from build123d import *

# Parameters (mm, degrees)
SKETCH_2_R      = 2
EXTRUDE_1_DEPTH = 2.5


with BuildPart() as part:
    # 草圖2 → 填料-伸長1 (new, symmetric)
    with BuildSketch(Plane.XY):
        with BuildLine():
            Line((7.226190238, -41.651673377), (4.413452329, 1.473554067))
            ThreePointArc((4.413452329, 1.473554067), (1.735862232, 4.991257537), (-2.546669656, 3.894149036))
            Line((-2.546669656, 3.894149036), (-41.492870765, -39.231078407))
            ThreePointArc((-41.492870765, -39.231078407), (-42.179656235, -43.536244411), (-38.524267862, -45.912010486))
            Line((-38.524267862, -45.912010486), (3.234671155, -45.912010486))
            ThreePointArc((3.234671155, -45.912010486), (6.153690549, -44.64684609), (7.226190238, -41.651673377))
        make_face()
        Circle(SKETCH_2_R, mode=Mode.SUBTRACT)
        with Locations((2.700997506, -41.412010486)):
            Circle(SKETCH_2_R, mode=Mode.SUBTRACT)
        with Locations((-37.399002494, -41.412010486)):
            Circle(SKETCH_2_R, mode=Mode.SUBTRACT)
    extrude(amount=EXTRUDE_1_DEPTH, both=True)


solid = part.part
Source: CAD feature listing. Evaluate the final solid. Frame: model axes, mm. Give positions to 0.01 mm unless a question says otherwise; leave off trailing zeros. Write each loop counter-clockwise with the first axis right and the second up, starting at its lowest first coordinate (ties: lowest second). Pieces come first, ordered by that corner, then holes. Notation, with made-up numbers: (57.25, 87.25) -> (106.25, 87.25) arc R32 cw to (106.25, 119.25) -> close; hole circle Ø6 at (22.5, 20.5). An arc over 180 degrees is marked (long way). Return JSON: item names as keys, results as strings. Group by question number.
1. Section C-C, the plane z = 1.2. Output: boundary loops of the cut face in (x, y).
2. Section D-D, the plane y = -34.5. Output: boundary loops of the cut face in (x, z).
3. Section B-B, the plane y = 0. Output: boundary loops of the cut face in (x, z).
4. Pin query (flat end, axial travel): pin 1 Ø3.5 at (x, y) = (-37.4, -41.41) entering from +Z; pin 2 Ø1.5 at (y, z) = (-27, -1) entering from +X. Return the tip coordinate at first contact, or that it passes through.
5. Material intervals for line 1 (Y direction, x = 3.5, z = -2.3); line 2 (Y direction, x = -39, z = -1.1); line 3 (X direction, y = -18, z = 1.15), sorted ascending. Write a range as from..to.
6. Section A-A, the plane x = 0. Output: boundary loops of the cut face in (y, z), then the cut area to 3 significant figures.
Determined:
{
 "1": {"outline": "(-41.49, -39.23) arc R4 ccw to (-38.52, -45.91) -> (3.23, -45.91) arc R4 ccw to (7.23, -41.65) -> (4.41, 1.47) arc R4 ccw to (-2.55, 3.89) -> close; hole circle Ø4 at (-37.4, -41.41); hole circle Ø4 at (0, 0); hole circle Ø4 at (2.7, -41.41)"},
 "2": {"outline": "(-37.22, -2.5) -> (6.76, -2.5) -> (6.76, 2.5) -> (-37.22, 2.5) -> close"},
 "3": {"outline": "(-6.06, -2.5) -> (-2, -2.5) -> (-2, 2.5) -> (-6.06, 2.5) -> close; (2, -2.5) -> (4.51, -2.5) -> (4.51, 2.5) -> (2, 2.5) -> close"},
 "4": {"pin 1": "passes through", "pin 2": "stops at x = 6.32"},
 "5": {"line 1": "y = -45.9..-43.25, -39.58..3.77", "line 2": "y = -45.88..-42.61, -40.21..-36.47", "line 3": "x = -22.32..5.68"},
 "6": {"outline": "(-45.91, -2.5) -> (-2, -2.5) -> (-2, 2.5) -> (-45.91, 2.5) -> close; (2, -2.5) -> (5.19, -2.5) -> (5.19, 2.5) -> (2, 2.5) -> close", "area": "236 mm2"}
}
